CAD build for the part. Positions are in the model's coordinates, mm. Face numbers are marked on the shaded views. A direction names the side the tool comes from. Coordinates: 2 decimals unless noted, no trailing zeros. Loops run counter-clockwise (first coordinate to the right, second up) from the corner with the lowest first, then second, coordinate; pieces in that order, holes last. Notation, with made-up numbers: (4, -35.5) -> (30, -35.5) arc R23 cw to (30, -2.5) -> close; hole circle Ø11 at (-7, -0.5). An arc over 180 degrees is marked (long way). Return JSON: item names as keys, results as strings. Group by question number.
(1) Probe L1, parallel to X at y = -9, z = 14.5; L2, parallel to X at y = -1, z = 27; L3, parallel to X at y = 4.25, z = 30. List the from-to ranges inside material, lowest first.
(2) Saw through at B-B on y = 2. Write the cut outline in (x, z).
(3) Tool access for the marked faces 1 and 2: list every direction of +Z, -Z, +X, -X, +Y, -Y with a clear straight run to the whole face (end or side of a thin tool).
(4) Mould opens along Z. For the marked faces 3, 4 and 5 say: pulls with the +Z half, pulls with the -Z half, needs draft (parallel to the pull), parting line crosses it, or undercut.
(5) Flat gauge pins, fed straight in: pin 1 Ø6 at (y, z) = (3.5, 18) entering from +X; pin 2 Ø6 at (x, y) = (55, -3.5) entering from -Z; pin 3 Ø5 at (x, y) = (59.35, 0) entering from -Z. Where does each tip first touch, or does it go through?
(6) Saw through at D-D on y = 8.75. Write the cut outline in (x, z).
(7) Saw through at C-C on y = -6. Write the cut outline in (x, z), then the cut area to 3 significant figures.
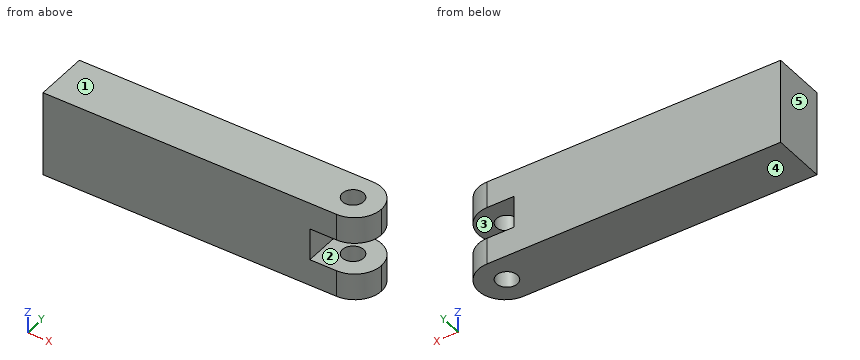
```python
from build123d import *

# Parameters (mm, degrees)
ESQUISSE2_W             = 100
ESQUISSE2_H             = 20
BOSS_EXTRU_1_DEPTH      = 32
ESQUISSE6_W             = 10
ESQUISSE6_H             = 20
BOSS_EXTRU_3_DEPTH      = 20
CONG_2_R                = 10
ESQUISSE7_R             = 3.96875
ENL_V_MAT_EXTRU_1_DEPTH = 78.614431648


with BuildPart() as part:
    # Esquisse2 → Boss.-Extru.1 (new body)
    with BuildSketch(Plane.XY):
        Rectangle(ESQUISSE2_W, ESQUISSE2_H)
    extrude(amount=BOSS_EXTRU_1_DEPTH)

    # Esquisse6 → Boss.-Extru.3 (add)
    with BuildSketch(Plane(origin=(50, 0, 0), x_dir=(0, 0, -1), z_dir=(1, 0, 0))):
        with Locations((-27, 0)):
            Rectangle(ESQUISSE6_W, ESQUISSE6_H)
        with Locations((-5, 0)):
            Rectangle(ESQUISSE6_W, ESQUISSE6_H)
    extrude(amount=BOSS_EXTRU_3_DEPTH)

    # Congé2
    cong_2_edges = [part.edges().sort_by_distance(p)[0] for p in [
        (70, -10, 27),
        (70, -10, 5),
        (70, 10, 5),
        (70, 10, 27),
    ]]
    fillet(cong_2_edges, radius=CONG_2_R - 0.0001)  # a hair under: the kernel refuses the full size

    # Esquisse7 → Enlèv. mat.-Extru.1 (cut, through all)
    with BuildSketch(Plane(origin=(0, 0, 0), x_dir=(-1, 0, 0), z_dir=(0, 0, -1))):
        with Locations((-59.35415424, 0)):
            Circle(ESQUISSE7_R)
    extrude(amount=-ENL_V_MAT_EXTRU_1_DEPTH, mode=Mode.SUBTRACT)


solid = part.part
```
Geometry results:
{
 "1": {"L1": "-50 to 50", "L2": "-50 to 55.51, 63.19 to 69.95", "L3": "-50 to 69.05"},
 "2": {"outline": "(-50, 0) -> (55.93, 0) -> (55.93, 10) -> (50, 10) -> (50, 22) -> (55.93, 22) -> (55.93, 32) -> (-50, 32) -> close; (62.78, 0) -> (69.8, 0) -> (69.8, 10) -> (62.78, 10) -> close; (62.78, 22) -> (69.8, 22) -> (69.8, 32) -> (62.78, 32) -> close"},
 "3": {"face 1": "+Z, +X, -X, +Y, -Y", "face 2": "+X, +Y, -Y"},
 "4": {"face 3": "undercut", "face 4": "pulls with the -Z half", "face 5": "needs draft"},
 "5": {"pin 1": "x = 50", "pin 2": "z = 0", "pin 3": "through"},
 "6": {"outline": "(-50, 0) -> (64.84, 0) -> (64.84, 10) -> (50, 10) -> (50, 22) -> (64.84, 22) -> (64.84, 32) -> (-50, 32) -> close"},
 "7": {"outline": "(-50, 0) -> (68, 0) -> (68, 10) -> (50, 10) -> (50, 22) -> (68, 22) -> (68, 32) -> (-50, 32) -> close", "area": "3,560 mm²"}
}
